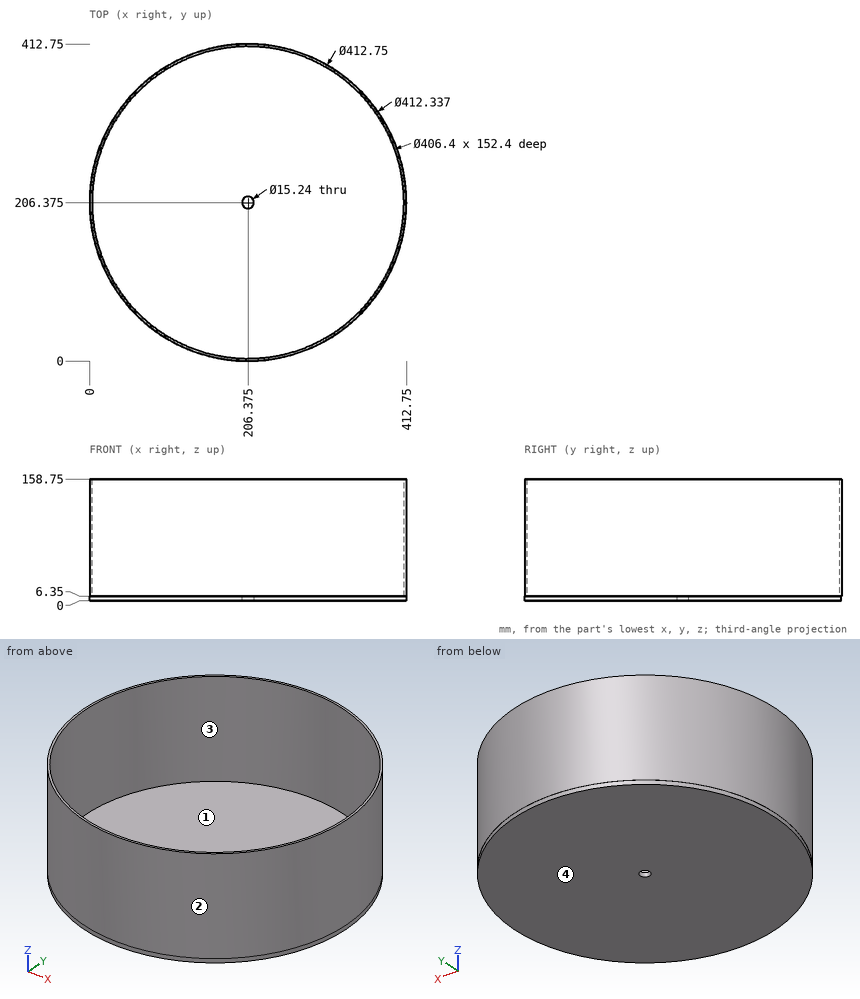
Answer from the drawing. Dimensions are ordinates in mm from the lowest x, y and z of the part. Give positions to 0.01 mm unless a question says otherwise; leave off trailing zeros. Answer as CSV lines item,"result".
Item 1: Determine the mould class of the marked faces 1, 2, 3 and 4 for opening direction Y: +Y half, -Y half, draft (parallel to the pull), parting line (faces both ways), or undercut.
Returned:
face 1,"undercut"
face 2,"parting line"
face 3,"undercut"
face 4,"draft"
Item 2: Consider line 1 (Z direction, x = 291, y = 332); line 2 (Y direction, x = 139, z = 47); line 3 (X direction, y = 58.5, z = 97). Determine where each line is inside the solid, lowest interval first. Write a range as [from, to].
Returned:
line 1,"z = [0, 6.35]"
line 2,"y = [11.31, 14.67], [398.08, 401.44]"
line 3,"x = [62.42, 67.01], [345.74, 350.33]"
Item 3: Each of these flat-tipped pins is pushed along its axis until it touches: pin 1 (12 mm diameter, centred on x = 180, z = 102.5, fed in from -Y); pin 2 (2 mm diameter, centred on x = 260, y = 285.5, fed in from -Z); pin 3 (1 mm diameter, centred on y = 167, z = 133.5, fed in from -X) (1 decimal); pin 4 (5 mm diameter, centred on x = 153, y = 95, fed in from +Z). Where does it stop, or does it pass through?
Returned:
pin 1,"stops at y = 1.01"
pin 2,"stops at z = 0"
pin 3,"stops at x = 3.7"
pin 4,"stops at z = 6.35"
